Geometry check sheet. Reference: the model listing, model coordinates, mm. Coordinates: 2 decimals unless noted, no trailing zeros. Order: outer loops, then holes, each group sorted by start corner. A loop starts at its lowest first (then second) coordinate and runs counter-clockwise, first axis right, second up. Notation, with made-up numbers: (4.5, 78) - (33.5, 78) arc R31 ccw to (33.5, 109) - close; hole circle Ø1 at (84.25, -3). An arc over 180 degrees is marked (long way). Put each result on its own line as item: value.
from build123d import *

# Parameters (mm, degrees)
BODY_SKETCH_W    = 95.89
BODY_SKETCH_H    = 90.17
BODY_DEPTH       = 1.6
HOLES_DEPTH      = 132.636169042
HOLES_DEPTH_BACK = 132.636169042
HOLES_SKETCH_R   = 1.7


with BuildPart() as part:
    # Body sketch → Body (new body)
    with BuildSketch(Plane.XY):
        with Locations((47.945, 45.085)):
            Rectangle(BODY_SKETCH_W, BODY_SKETCH_H)
    extrude(amount=BODY_DEPTH)

    # Holes sketch → Holes (cut, two sides: drawn at the far end of the back side and taken through both)
    with BuildSketch(Plane.XY.offset(-HOLES_DEPTH_BACK)):
        with Locations((5.08, 5.08)):
            Circle(HOLES_SKETCH_R)
        with Locations((90.81, 5.08)):
            Circle(HOLES_SKETCH_R)
        with Locations((5.08, 85.09)):
            Circle(HOLES_SKETCH_R)
        with Locations((90.81, 85.09)):
            Circle(HOLES_SKETCH_R)
    extrude(amount=HOLES_DEPTH + HOLES_DEPTH_BACK, mode=Mode.SUBTRACT)


solid = part.part
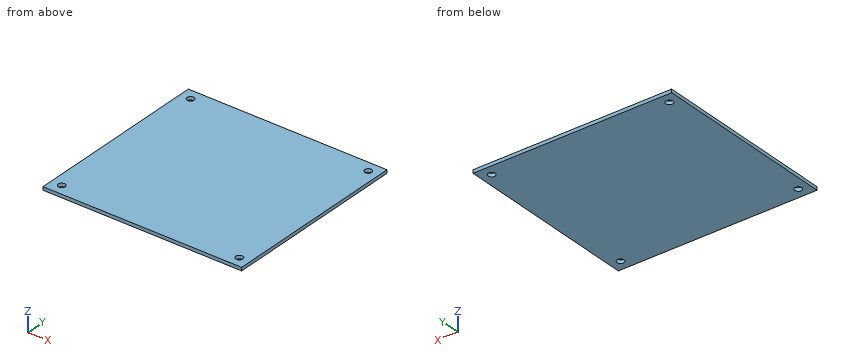
Q1. Thickness scan on L1, parallel to X at y = 5.08, z = 0.7; L2, parallel to Y at x = 90.81, z = 0.8; L3, parallel to X at y = 85.5, z = 1.35. Record the ranges inside material, lowest first. Write a range as [from, to].
Answer block:
L1: x = [0, 3.38], [6.78, 89.11], [92.51, 95.89]
L2: y = [0, 3.38], [6.78, 83.39], [86.79, 90.17]
L3: x = [0, 3.43], [6.73, 89.16], [92.46, 95.89]
Q2. Section check B-B on y = 85.09. Record the boundary of the cut face in (x, z), then the cut area to 3 significant figures.
Answer block:
outline: (0, 0) - (3.38, 0) - (3.38, 1.6) - (0, 1.6) - close; (6.78, 0) - (89.11, 0) - (89.11, 1.6) - (6.78, 1.6) - close; (92.51, 0) - (95.89, 0) - (95.89, 1.6) - (92.51, 1.6) - close
area: 143 mm^2
Q3. Section check A-A on x = 90.81. Record the boundary of the cut face in (y, z), then the cut area to 3 significant figures.
Answer block:
outline: (0, 0) - (3.38, 0) - (3.38, 1.6) - (0, 1.6) - close; (6.78, 0) - (83.39, 0) - (83.39, 1.6) - (6.78, 1.6) - close; (86.79, 0) - (90.17, 0) - (90.17, 1.6) - (86.79, 1.6) - close
area: 133 mm^2
